Could you check a few things on this drawing? It's one solid part, dimensions in mm from its lowest x, y, z. Give positions to 0.01 mm unless a question says otherwise; leave off trailing zeros. Order: outer loops, then holes, each group sorted by start corner. A loop starts at its lowest first (then second) coordinate and runs counter-clockwise, first axis right, second up.
(1) Imagine slicing it at A-A, the plane y = 33. Write out the boundary of the cut face in (x, z).
(2) If we mould it in two halves opening along Z, with no side actions, what happens to the marked faces 1 and 2? For each: released by +Z, released by -Z, zero draft, split by the parting line, or undercut.
(3) Will these pins go through, and if not, where does the flat tip stop? pin 1 (3 mm diameter, centred on y = 18, z = 20, fed in from +X); pin 2 (6 mm diameter, centred on x = 8, y = 42.5, fed in from +Z); pin 3 (5 mm diameter, centred on y = 20.5, z = 13, fed in from -X).
(4) If I drill on probe 1 along X at (y, z) = (5, 16); probe 2 along X at (y, z) = (22.5, 26.5), over which ranges is the centre line in solid material (lowest first)?
(5) Imagine slicing it at B-B, the plane y = 22. Write out the boundary of the cut face in (x, z), then the cut area to 3 significant figures.
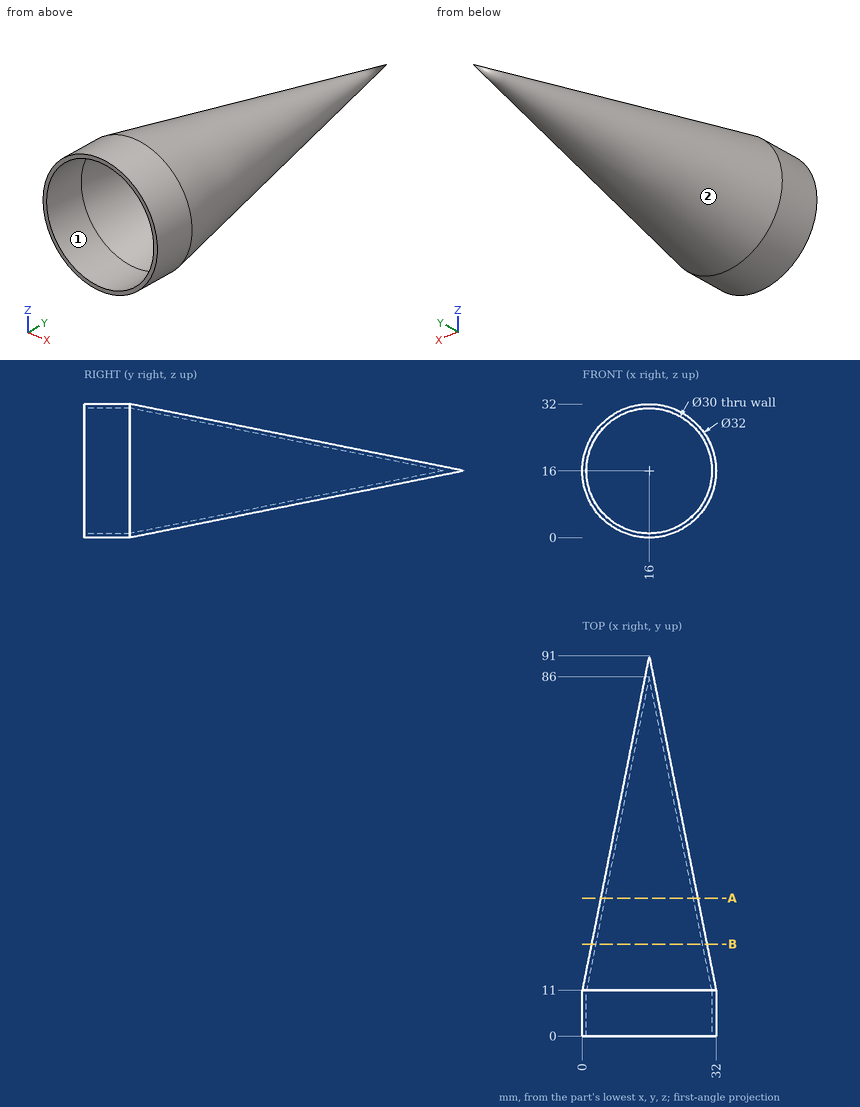
Answer block:
1. outline: circle Ø23.2 at (16, 16); hole circle Ø21.2 at (16, 16)
2. face 1: undercut
2. face 2: split by the parting line
3. pin 1: stops at x = 30.52
3. pin 2: stops at z = 24.44
3. pin 3: stops at x = 1.57
4. probe 1: x = 0 to 1, 31 to 32
4. probe 2: x = 7.2 to 8.86, 23.14 to 24.8
5. outline: circle Ø27.6 at (16, 16); hole circle Ø25.6 at (16, 16)
5. area: 83.6 mm2
